Model file for the job. Use its own axes, mm. A direction names the side the tool comes from. Give positions to 0.01 mm unless a question says otherwise; leave off trailing zeros. Write each loop counter-clockwise with the first axis right and the second up, starting at its lowest first coordinate (ties: lowest second). Pieces come first, ordered by that corner, then holes. Notation, with made-up numbers: (-3.75, 47.25) - (2.25, 47.25) arc R11 cw to (2.25, 68.25) - close; hole circle Ø8 at (61, -32.75). An arc over 180 degrees is marked (long way). One line per item, written item: value. Start each with the question number.
(1) Probe L1, parallel to Y at x = 10.16, z = 2.4; L2, parallel to X at y = 16.75, z = 0.2; L3, parallel to Y at x = 19, z = 0.8. List the from-to ranges inside material, lowest first.
(2) Cut at A-A, the plane x = 87.5. List the corners of the cut face in (y, z), and give its area (3 significant figures).
(3) Cut at C-C, the plane x = 10.16. List the corners of the cut face in (y, z), and give its area (3 significant figures).
(4) 3-axis set-ups, long thin cutter, end or side, ignore diameter. For faces 1 (the face through (91.999, 1, 4)), 2 (the face through (61, 2.54, 3)), 3 (the face through (41, 17, 5.436)), 4 (the face through (98, 16, 1.27)): which of +Z, -Z, +X, -X, +Y, -Y reach the whole face in a straight line?
(5) Cut at B-B, the plane y = 8.89. List the corners of the cut face in (x, z), and give its area (3 significant figures).
(6) Drop flat-ended pins along their axis: P1, Ø3, axis at y = 1.5, z = 3.5, coming from the +X side; P2, Ø2, axis at x = 98.5, y = 17, coming from the -Z side. Give the stop position or say it passes through.
from build123d import *

# Parameters (mm, degrees)
F0_W      = 117.3988
F0_H      = 17.78
F1_DEPTH  = 5.4356
F2_W      = 88.9
F2_H      = 12.7
F3_DEPTH  = 25.4
F4_W      = 11.43
F4_H      = 12.7
F5_DEPTH  = 3.81
F7_DEPTH  = 169
F8_R      = 1.24968
F9_DEPTH  = 5.4356
F10_W     = 5.08
F10_H     = 2.54
F11_DEPTH = 1.27


# Not quite as in the source:
# - an extrude ends at something that could not be found from the text; its depth is read off the source's solid


with BuildPart() as f1:
    # F0 (on Top) → F1 (new body)
    with BuildSketch(Plane.XY):
        with Locations((58.6994, 8.89)):
            Rectangle(F0_W, F0_H)
    extrude(amount=F1_DEPTH)

    # F2 (on face) → F3 (cut)
    with BuildSketch(Plane.XY.offset(5.4356)):
        with Locations((61.5188, 8.89)):
            Rectangle(F2_W, F2_H)
    extrude(amount=-F3_DEPTH, mode=Mode.SUBTRACT)

    # F4 (on face) → F5 (cut)
    with BuildSketch(Plane.XY.offset(5.4356)):
        with Locations((111.6838, 8.89)):
            Rectangle(F4_W, F4_H)
    extrude(amount=-F5_DEPTH, mode=Mode.SUBTRACT)

    # F6 (on face) → F7 (cut, through all)
    with BuildSketch(Plane.XY.offset(1.6256)):
        Polygon((105.9688, 2.54), (105.9688, 15.24), (91.9988, 15.24), (91.9988, 0), (117.3988, 0), (117.3988, 2.54), align=None)
    extrude(amount=F7_DEPTH, mode=Mode.SUBTRACT)

    # F8 (on face) → F9 (cut, through all)
    with BuildSketch(Plane.XY.offset(5.4356)):
        with Locations((10.16, 8.89)):
            Circle(F8_R)
    extrude(amount=-F9_DEPTH, mode=Mode.SUBTRACT)

    # F10 (on face) → F11 (cut)
    with BuildSketch(Plane(origin=(0, 0, 0), x_dir=(1, 0, 0), z_dir=(0, 0, -1))):
        with Locations((98.3488, -16.51)):
            Rectangle(F10_W, F10_H)
        Polygon((95.8088, -15.24), (100.8888, -15.24), (105.9688, -15.24), (105.9688, -2.54), (17.0688, -2.54), (17.0688, -15.24), align=None)
    extrude(amount=-F11_DEPTH, mode=Mode.SUBTRACT)


solid = f1.part
Answers follow:
1. L1: y = 0 to 7.64, 10.14 to 17.78
1. L2: x = 0 to 95.81, 100.89 to 117.4
1. L3: y = 0 to 2.54, 15.24 to 17.78
2. outline: (0, 0) - (2.54, 0) - (2.54, 5.44) - (0, 5.44) - close; (15.24, 0) - (17.78, 0) - (17.78, 5.44) - (15.24, 5.44) - close
2. area: 27.6 mm²
3. outline: (0, 0) - (7.64, 0) - (7.64, 5.44) - (0, 5.44) - close; (10.14, 0) - (17.78, 0) - (17.78, 5.44) - (10.14, 5.44) - close
3. area: 83.1 mm²
4. face 1: +Z, +X, -Y
4. face 2: +Z, -Z
4. face 3: +Z, +X, -X, +Y, -Y
4. face 4: -Z, +Y
5. outline: (0, 0) - (8.91, 0) - (8.91, 5.44) - (0, 5.44) - close; (11.41, 0) - (17.07, 0) - (17.07, 5.44) - (11.41, 5.44) - close; (105.97, 0) - (117.4, 0) - (117.4, 1.63) - (105.97, 1.63) - close
5. area: 97.8 mm²
6. P1: stops at x = 92
6. P2: stops at z = 1.27
